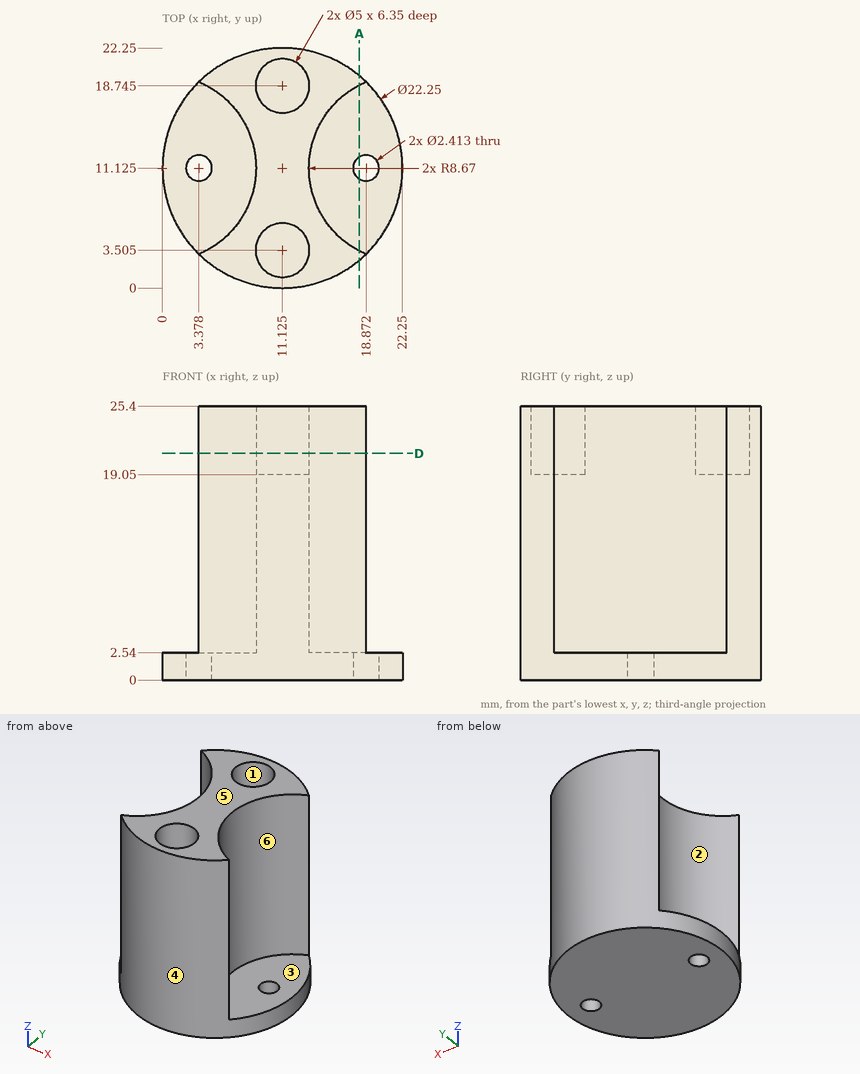
Can you work these out from the drawing? Everything is in mm from the part's minimum corner. A direction names the side the tool comes from. Coordinates: 2 decimals unless noted, no trailing zeros. Order: outer loops, then holes, each group sorted by start corner. A loop starts at its lowest first (then second) coordinate and runs counter-clockwise, first axis right, second up. Notation, with made-up numbers: (16.5, 64.25) -> (33.5, 64.25) arc R30 cw to (33.5, 96.25) -> close; hole circle Ø8 at (66.5, 32.25). An arc over 180 degrees is marked (long way). Use one line per item in the form item = value.
Q1. We'd pull the mould along Y, two halves only. Please class the marked faces 4, 5 and 6: released by +Y, released by -Y, zero draft, split by the parting line, or undercut.
From the geometry:
face_4 = split by the parting line
face_5 = zero draft
face_6 = undercut
Q2. Imagine slicing it at D-D, the plane z = 21. Give the number of separate pieces and of enclosed holes in the cut face, then the cut area to 3 significant figures.
From the geometry:
separate_pieces = 1
enclosed_holes = 2
area = 153 mm²
Q3. Imagine slicing it at A-A, the plane x = 18.25. List the corners of the cut face in (y, z) for me.
From the geometry:
outline = (2.58, 0) -> (10.09, 0) -> (10.09, 2.54) -> (3.43, 2.54) -> (3.43, 25.4) -> (2.58, 25.4) -> close; (12.16, 0) -> (19.67, 0) -> (19.67, 25.4) -> (18.82, 25.4) -> (18.82, 2.54) -> (12.16, 2.54) -> close
Q4. Which directions (+Z, -Z, +X, -X, +Y, -Y) give clear straight access to the entire face, cutting with the end or side of a thin tool? Please do the marked faces 1, 2 and 3.
From the geometry:
face_1 = +Z
face_2 = +Z, -X
face_3 = +Z, +X
Q5. Will these pins go through, and if not, where does the flat tip stop? P1, Ø1.4, axis at x = 18.87, y = 11.13, coming from the -Z side (3 decimals); P2, Ø6, axis at x = 20, z = 17, coming from the -Y side; P3, Ø4, axis at x = 5.5, z = 15.5, coming from the -Y side; P4, Ø8, axis at y = 6, z = 15.5, coming from the +X side.
From the geometry:
P1 = through
P2 = 1.68
P3 = 0.61
P4 = 18.87
Q6. I need wall thicknesses on L1, parallel to Y at x = 11.5, z = 7; L2, parallel to X at y = 4, z = 24 (1 decimal); L3, parallel to X at y = 5.25, z = 20 (1 decimal). Which ranges of each line are inside material? Lowest first, please.
From the geometry:
L1 = 0.01 to 22.24
L2 = 4.9 to 8.7, 13.6 to 17.3
L3 = 6.4 to 9.3, 12.9 to 15.9
